Verification items for the finished model (mm, model axes). A direction names the side the tool comes from. Coordinates: 2 decimals unless noted, no trailing zeros. Loops run counter-clockwise (first coordinate to the right, second up) from the corner with the lowest first, then second, coordinate; pieces in that order, holes last. Notation, with made-up numbers: M -9.5,20 L 10.5,20 A28 cw 10.5,54 Z; hole C -11.75,87.25 d3. An arc over 180 degrees is marked long. Write item = value, one per line. Start each with the question number.
```python
from build123d import *

# Parameters (mm, degrees)
SKETCH1_R           = 11.55
BOSS_EXTRUDE1_DEPTH = 33.22
BOSS_EXTRUDE2_DEPTH = 6.1
SKETCH3_R           = 2.4
CUT_EXTRUDE1_DEPTH  = 8.3
CHAMFER1_SIZE       = 0.5
SKETCH4_R           = 2.45
BOSS_EXTRUDE3_DEPTH = 4.7
BOSS_EXTRUDE4_START = 6.793009
BOSS_EXTRUDE4_DEPTH = 0.706991


with BuildPart() as part:
    # Sketch1 → Boss-Extrude1 (new body)
    with BuildSketch(Plane.XY):
        Circle(SKETCH1_R)
    extrude(amount=BOSS_EXTRUDE1_DEPTH)

    # Sketch2 → Boss-Extrude2 (add)
    with BuildSketch(Plane.XY.offset(33.22)):
        with BuildLine():
            Line((5, 3.234505372), (5, -3.234505372))
            ThreePointArc((5, -3.234505372), (0, -5.955), (-5, -3.234505372))
            Line((-5, -3.234505372), (-5, 3.234505372))
            ThreePointArc((-5, 3.234505372), (0, 5.955), (5, 3.234505372))
        make_face()
    extrude(amount=BOSS_EXTRUDE2_DEPTH)

    # Sketch3 → Cut-Extrude1 (cut)
    with BuildSketch(Plane.XY.offset(39.32)):
        Circle(SKETCH3_R)
    extrude(amount=-CUT_EXTRUDE1_DEPTH, mode=Mode.SUBTRACT)

    # Chamfer1
    chamfer1_edges = [part.edges().sort_by_distance(p)[0] for p in [
        (-2.4, 0, 39.32),
    ]]
    chamfer(chamfer1_edges, length=CHAMFER1_SIZE)

    # Sketch4 → Boss-Extrude3 (add)
    with BuildSketch(Plane(origin=(0, 0, 0), x_dir=(-1, 0, 0), z_dir=(0, 0, -1))):
        with BuildLine():
            Line((4.5, 2.179449472), (4.5, -2.179449472))
            ThreePointArc((4.5, -2.179449472), (0, -5), (-4.5, -2.179449472))
            Line((-4.5, -2.179449472), (-4.5, 2.179449472))
            ThreePointArc((-4.5, 2.179449472), (0, 5), (4.5, 2.179449472))
        make_face()
        Circle(SKETCH4_R, mode=Mode.SUBTRACT)
    extrude(amount=BOSS_EXTRUDE3_DEPTH)

    # Sketch5 → Boss-Extrude4 (add)
    with BuildSketch(Plane(origin=(4.5, 0, 0), x_dir=(0, 0, -1), z_dir=(1, 0, 0)).offset(BOSS_EXTRUDE4_START)):
        Polygon((-24.291547622, 0), (-22.281436224, 2.422902131), (-22.281436224, 0.987108276), (-18.60765225, 0.987108276), (-18.60765225, -0.987108276), (-22.281436224, -0.987108276), (-22.281436224, -2.422902131), align=None)
    extrude(amount=BOSS_EXTRUDE4_DEPTH)


solid = part.part
```
Q1. Sectioned sample at B-B on z = 32.5. Record the cut outline in (x, y), plus the area to 3 significant figures.
Q2. Scan lines: L1, parallel to Y at x = 0, z = 33; L2, parallel to Y at x = 0, z = 36.75 (3 decimals); L3, parallel to Z at x = 5.75, y = 6.5. Record each from-to range of solid material in increasing order. Write a range as [from, to].
Q3. Sectioned sample at A-A on x = 0. Record the cut outline in (y, z) (3 decimals).
Q4. Set-up check for faces 4 (the face through (-5.3, 0.2, 33.22)), 5 (the face through (5, 0, 0)), 6 (the face through (11.72, 1.194, 23.301)), 7 (the face through (-4.5, 0, -2)), 8 (the face through (-5, 0, 36)): record each of +Z, -Z, +X, -X, +Y, -Y from which the full face is reachable in a straight line by a thin tool's end or side.
Q5. Gauge pin test, flat ends, axial feed: pin 1 (4.5 mm diameter, centred on x = 0, y = 0, fed in from +Z); pin 2 (0.8 mm diameter, centred on x = 11.5, y = 2, fed in from -Z); pin 3 (5 mm diameter, centred on y = 1.5, z = 35.5, fed in from +X). Record the tip position at first contact, or that the pin passes through.
Q6. Sectioned sample at C-C on y = -4.5. Record the cut outline in (x, z).
Q7. Mould release check, pull along Y, two halves, no side actions. Record for faces 1 (the face through (11.72, -1.23, 23.27)), 2 (the face through (0, 5, -2)), 3 (the face through (0.5, -2.4, -2.3)): +Y half, -Y half, draft (parallel to the pull), parting line (faces both ways), or undercut.
Q8. Sectioned sample at D-D on z = 3.5. Record the cut outline in (x, y), plus the area to 3 significant figures.
Solutions:
q1.outline = C 0,0 d23.1; hole C 0,0 d4.8
q1.area = 401 mm²
q2.L1 = [-11.55, -2.4], [2.4, 11.55]
q2.L2 = [-5.955, -2.4], [2.4, 5.955]
q2.L3 = [0, 33.22]
q3.outline = M -11.55,0 L -5,0 L -5,-4.7 L -2.45,-4.7 L -2.45,0 L 2.45,0 L 2.45,-4.7 L 5,-4.7 L 5,0 L 11.55,0 L 11.55,33.22 L 5.955,33.22 L 5.955,39.32 L 2.9,39.32 L 2.4,38.82 L 2.4,31.02 L -2.4,31.02 L -2.4,38.82 L -2.9,39.32 L -5.955,39.32 L -5.955,33.22 L -11.55,33.22 Z
q4.face_4 = +Z
q4.face_5 = -Z
q4.face_6 = +Z, +X, +Y
q4.face_7 = -Z, -X, +Y, -Y
q4.face_8 = +Z, -X, +Y, -Y
q5.pin_1 = 31.02
q5.pin_2 = 0
q5.pin_3 = 11.54
q6.outline = M -10.64,0 L -2.18,0 L -2.18,-4.7 L 2.18,-4.7 L 2.18,0 L 10.64,0 L 10.64,33.22 L 3.9,33.22 L 3.9,39.32 L -3.9,39.32 L -3.9,33.22 L -10.64,33.22 Z
q7.face_1 = -Y half
q7.face_2 = +Y half
q7.face_3 = undercut
q8.outline = C 0,0 d23.1
q8.area = 419 mm²
